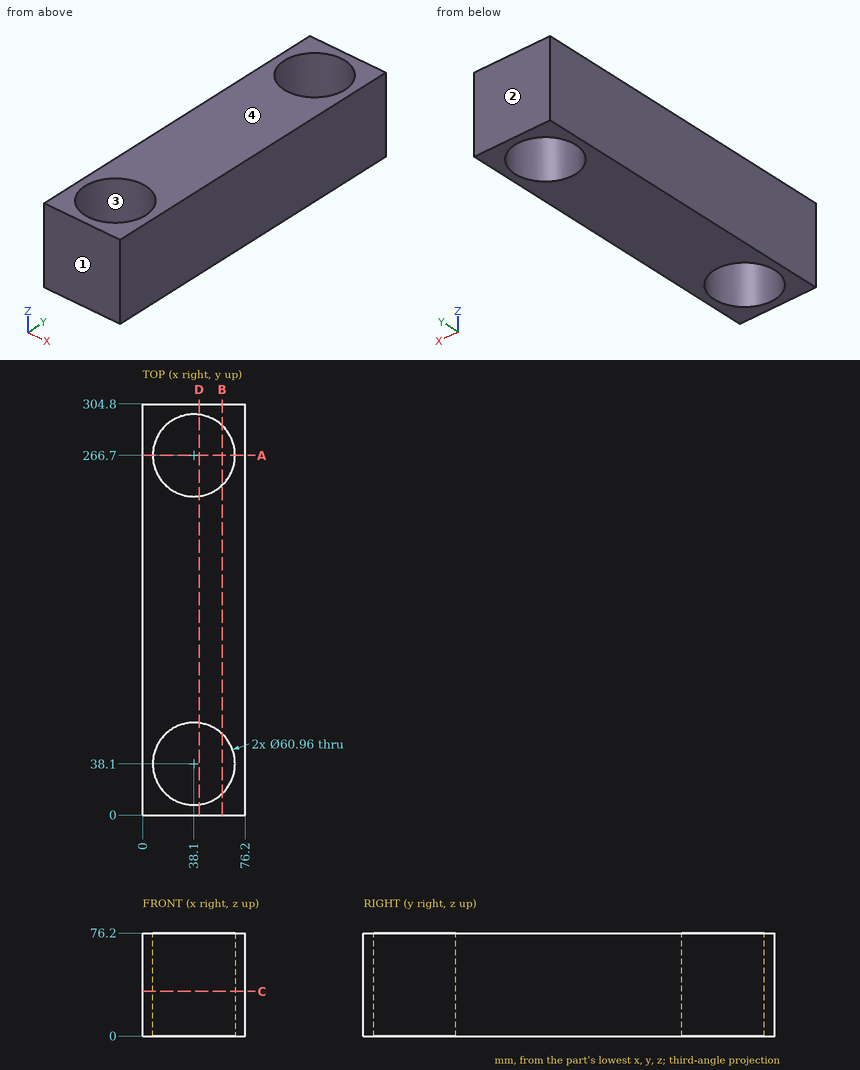
Geometry: see drawing. Coordinates: mm, zero at the bounding-box minimum. Coordinates: 2 decimals unless noted, no trailing zeros. Order: outer loops, then holes, each group sorted by start corner. A loop starts at its lowest first (then second) coordinate and runs counter-clockwise, first axis right, second up. Notation, with made-up numbers: M 32.25,75.5 L 85.25,75.5 A37 cw 85.25,113.5 Z; hole C 86,23.25 d11. An arc over 180 degrees is marked long. Answer in a Markdown table with one row per item. Add a question column.
Q1. Contact query for flat-ended pins moving along their axis: P1, Ø6, axis at x = 39.5, y = 63.5, coming from the +Z side; P2, Ø5, axis at x = 61, z = 10, coming from the -Y side. Output: stop coordinate, or through.
Q2. Section query A-A on y = 266.7. Return the cut outline in (x, z).
Q3. Line query: L1, parallel to Y at x = 38.1, z = 45; L2, parallel to X at y = 266, z = 42; L3, parallel to Y at x = 40, z = 4. Output: solid intervals per line, ascending.
Q4. Section query B-B on x = 59. Return the cut outline in (y, z), and give its area (3 significant figures).
Q5. Section query C-C on z = 33. Return the cut outline in (x, y), and give its area (3 significant figures).
Q6. Mould query, pull axis Y, two halves, no side actions, for the marked faces 1, 2, 3 and 4. Classes: released by +Y, released by -Y, zero draft, split by the parting line, or undercut.
Q7. Section query D-D on x = 42. Return the cut outline in (y, z), and give its area (3 significant figures).
Completed:
| question | item | result |
|---|---|---|
| 1 | P1 | passes through |
| 1 | P2 | stops at y = 0 |
| 2 | outline | M 0,0 L 7.62,0 L 7.62,76.2 L 0,76.2 Z; M 68.58,0 L 76.2,0 L 76.2,76.2 L 68.58,76.2 Z |
| 3 | L1 | y = 0 to 7.62, 68.58 to 236.22, 297.18 to 304.8 |
| 3 | L2 | x = 0 to 7.63, 68.57 to 76.2 |
| 3 | L3 | y = 0 to 7.68, 68.52 to 236.28, 297.12 to 304.8 |
| 4 | outline | M 0,0 L 15.91,0 L 15.91,76.2 L 0,76.2 Z; M 60.29,0 L 244.51,0 L 244.51,76.2 L 60.29,76.2 Z; M 288.89,0 L 304.8,0 L 304.8,76.2 L 288.89,76.2 Z |
| 4 | area | 16,500 mm2 |
| 5 | outline | M 0,0 L 76.2,0 L 76.2,304.8 L 0,304.8 Z; hole C 38.1,38.1 d60.96; hole C 38.1,266.7 d60.96 |
| 5 | area | 17,400 mm2 |
| 6 | face 1 | released by -Y |
| 6 | face 2 | released by +Y |
| 6 | face 3 | undercut |
| 6 | face 4 | zero draft |
| 7 | outline | M 0,0 L 7.87,0 L 7.87,76.2 L 0,76.2 Z; M 68.33,0 L 236.47,0 L 236.47,76.2 L 68.33,76.2 Z; M 296.93,0 L 304.8,0 L 304.8,76.2 L 296.93,76.2 Z |
| 7 | area | 14,000 mm2 |
